Here's how the part is built. I have some questions about the finished solid (model axes, mm). Face numbers are marked on the shaded views. A direction names the side the tool comes from. Coordinates: 2 decimals unless noted, no trailing zeros. Write each loop counter-clockwise with the first axis right and the second up, starting at its lowest first coordinate (ties: lowest second). Pieces come first, ordered by that corner, then holes. Notation, with made-up numbers: M 46.25,63 L 59.25,63 A13 cw 59.25,79 Z; hole C -13,18 d4. An arc over 180 degrees is marked long. Use one line per item in the form item = value. Start each with the question number.
1. I want a section at C-C, the plane y = 52. List the corners of the cut face in (x, z) for me.
2. I want a section at A-A, the plane z = 6. List the corners of the cut face in (x, y) for me, plus the area to 3 significant figures.
3. On a 3-axis mill with a long thin cutter (end or side, diameter ignored), from which of +Z, -Z, +X, -X, +Y, -Y can I reach the whole of each face in a straight line? I mean the marked faces 1, 2 and 3. Say none if no direction works.
4. Thinking about a two-plate mould opening in Y: for the marked faces 4, 5, 6 and 7, which applies, released by +Y, released by -Y, zero draft, split by the parting line, or undercut?
5. I want a section at B-B, the plane x = 133.5. List the corners of the cut face in (y, z) for me, plus the area to 3 significant figures.
6. I'm going to push flat-ended pins straight in: pin 1 Ø6 at (y, z) = (38.5, 7.5) entering from +X; pin 2 Ø3 at (y, z) = (61, 8.5) entering from -X; pin 3 Ø10 at (x, y) = (145.5, 16) entering from -Z. Where does each tip first touch, or does it pass through?
7. I want a section at D-D, the plane y = 11. List the corners of the cut face in (x, z) for me.
8. Please list where these lines run through material, in increasing order: line 1 along Y through (x, z) = (160.5, 13.5); line 2 along Y through (x, z) = (28, 6.75); line 3 along X through (y, z) = (52.5, 10). Write a range as [from, to].
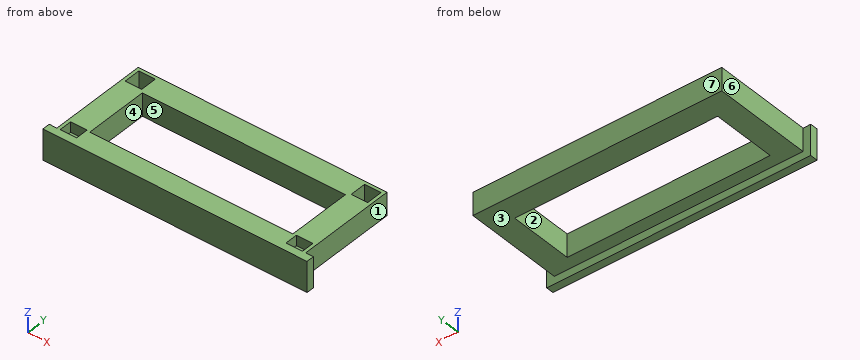
Autodesk Inventor part; units mm, degrees
ref_plane "YZ Plane" through (0, 0, 0) normal (1, 0, 0) x (0, 1, 0)
ref_plane "XZ Plane" through (0, 0, 0) normal (0, 1, 0) x (-1, 0, 0)
ref_plane "XY Plane" through (0, 0, 0) normal (0, 0, 1) x (1, 0, 0)
sketch "Sketch1" plane through (0, 0, 0) normal (0, 0, 1) x (1, 0, 0)
  line L0 (0, 0) -> (0, 70)
  line L1 (0, 70) -> (163, 70)
  line L2 (163, 70) -> (163, 0)
  line L3 (163, 0) -> (0, 0)
  line L4 (0, 70) -> (15, 70)
  line L5 (15, 55) -> (15, 13)
  line L6 (0, 70) -> (0, 55)
  line L7 (15, 55) -> (148, 55)
  line L8 (163, 70) -> (148, 70)
  line L9 (148, 55) -> (148, 13)
  line L10 (163, 0) -> (163, 13)
  line L11 (148, 13) -> (15, 13)
  dimension "d0" = 70
  dimension "d1" = 163
  dimension "d2" = 15
  dimension "d3" = 15
  dimension "d4" = 15
  dimension "d5" = 13
extrude "Extrusion1" add sketch "Sketch1" along normal blind 15
sketch "Sketch2" plane through (0, 0, 0) normal (0, 0, -1) x (-1, 0, 0)
  line L0 (-163, 0) -> (-163, 70)
  line L1 (-163, 0) -> (-163, 5)
  line L2 (-163, 5) -> (0, 5)
  line L3 (0, 0) -> (-163, 0)
  line L4 (-163, 0) -> (0, 0)
  line L5 (-163, 0) -> (0, 0)
  line L6 (0, 0) -> (0, 5)
  line L7 (0, 5) -> (-163, 5)
  line L8 (-163, 5) -> (-163, 0)
  dimension "d8" = 5
extrude "Extrusion2" add sketch "Sketch2" along normal blind 5
sketch "Sketch3" plane through (163, 0, 15) normal (1, 0, 0) x (0, 0, -1)
  line L0 (20, 5) -> (20, 0)
  line L1 (0, 0) -> (20, 0)
  line L2 (20, 0) -> (20, 5)
  line L3 (20, 5) -> (0, 5)
  line L4 (0, 5) -> (0, 0)
  point P0 (15, 0)
extrude "Extrusion3" add sketch "Sketch3" along normal blind 5
ref_plane "Work Plane1" through (81.5, 70, 15) normal (1, 0, 0) x (0, 0, -1)
mirror "Mirror1" about plane through (81.5, 70, 15) normal (1, 0, 0) of "Extrusion3"
sketch "Sketch4" plane through (0, 0, 15) normal (0, 0, 1) x (1, 0, 0)
  line L0 (163, 70) -> (0, 70)
  line L1 (15, 55) -> (148, 55)
  line L2 (0, 70) -> (2.5003, 67.4997) construction
  line L3 (2.5003, 67.4997) -> (2.5003, 57.4997)
  line L4 (2.5003, 57.4997) -> (12.5003, 57.4997)
  line L5 (12.5003, 57.4997) -> (12.5003, 67.4997)
  line L6 (12.5003, 67.4997) -> (2.5003, 67.4997)
  line L7 (148, 13) -> (15, 13)
  line L8 (15, 13) -> (12.5, 13) construction
  line L9 (12.5, 13) -> (2.5, 13)
  line L10 (2.5, 13) -> (2.5, 5.5)
  line L11 (2.5, 5.5) -> (12.5, 5.5)
  line L12 (12.5, 5.5) -> (12.5, 13)
  line L13 (2.1, 13.4) -> (12.9, 13.4)
  line L14 (12.9, 13.4) -> (12.9, 5.1)
  line L15 (12.9, 5.1) -> (2.1, 5.1)
  line L16 (2.1, 5.1) -> (2.1, 13.4)
  line L17 (12.9003, 57.0997) -> (2.1003, 57.0997)
  line L18 (2.1003, 57.0997) -> (2.1003, 67.8997)
  line L19 (2.1003, 67.8997) -> (12.9003, 67.8997)
  line L20 (12.9003, 67.8997) -> (12.9003, 57.0997)
  point P0 (0, 0)
  dimension "d13" = 3.536
  dimension "d14" = 10
  dimension "d15" = 10
  dimension "d16" = 10
  dimension "d17" = 2.5
  dimension "d18" = 10
  dimension "d19" = 7.5
  dimension "d20" = 10
  dimension "d22" = 0.4
  dimension "d23" = 0.4
extrude "Extrusion4" cut sketch "Sketch4" against normal blind 6.7 contours L12 L11 L10 L9 | L13 L14 L15 L16
extrude "Extrusion5" cut sketch "Sketch4" against normal blind 14.2 contours L6 L5 L4 L3 | L17 L18 L19 L20
mirror "Mirror2" about plane through (81.5, 70, 15) normal (1, 0, 0) of "Extrusion4", "Extrusion5"
properties part number "Front Facing Beam Support"
Answer list:
q1.outline = M 0,0 L 15,0 L 15,15 L 0,15 Z; M 148,0 L 163,0 L 163,15 L 148,15 Z
q2.outline = M -5,0 L 168,0 L 168,5 L 163,5 L 163,70 L 0,70 L 0,5 L -5,5 Z; hole M 2.1,57.1 L 12.9,57.1 L 12.9,67.9 L 2.1,67.9 Z; hole M 15,13 L 148,13 L 148,55 L 15,55 Z; hole M 150.1,57.1 L 160.9,57.1 L 160.9,67.9 L 150.1,67.9 Z
q2.area = 5,640 mm²
q3.face_1 = +Z, -Z, +X, +Y
q3.face_2 = +Z, -Z
q3.face_3 = -Z, +X, -X, +Y
q4.face_4 = undercut
q4.face_5 = undercut
q4.face_6 = zero draft
q4.face_7 = released by +Y
q5.outline = M 0,-5 L 5,-5 L 5,0 L 13,0 L 13,15 L 0,15 Z; M 55,0 L 70,0 L 70,15 L 55,15 Z
q5.area = 445 mm²
q6.pin_1 = 163
q6.pin_2 = 0
q6.pin_3 = 0
q7.outline = M 0,0 L 163,0 L 163,15 L 160.9,15 L 160.9,8.3 L 150.1,8.3 L 150.1,15 L 12.9,15 L 12.9,8.3 L 2.1,8.3 L 2.1,15 L 0,15 Z
q8.line_1 = [0, 5.1], [13.4, 57.1], [67.9, 70]
q8.line_2 = [0, 13], [55, 70]
q8.line_3 = [0, 15], [148, 163]
